Work out the finished part from the listing and answer in its coordinate system (mm). A direction names the side the tool comes from. Coordinates: 2 decimals unless noted, no trailing zeros. Order: outer loops, then holes, each group sorted by start corner. A loop starts at its lowest first (then second) coordinate and runs counter-clockwise, first axis right, second up. Notation, with made-up numbers: M 10,-15 L 26,-15 A23 ccw 26,19 Z; hole C 52,75.25 d3. An arc over 180 degrees is marked long. Answer in a Markdown table with one row per item. Add a question column.
Item 1: The part is cut by section B-B (z = 4). Write down the section's boundary in (x, y).
Item 2: Which of the six approach directions +Z, -Z, +X, -X, +Y, -Y give full straight-line access (tool end or side, diameter ignored) to faces 1 (the face through (-15.54, -11.7, 11.1)), 2 (the face through (0, -36, 3)), 3 (the face through (0, -8, 3))?
Item 3: The part is cut by section D-D (z = 13.25). Write down the section's boundary in (x, y).
Item 4: The mould has two halves that part along Y. Classify faces 4 (the face through (-7, -10.32, 10)), 5 (the face through (-5.881, -9.334, 11.236)), 6 (the face through (2, -15.32, 6)): released by +Y, released by -Y, zero draft, split by the parting line, or undercut.
Item 5: Consider line 1 (Y direction, x = -12.85, z = 11.15); line 2 (Y direction, x = -6.15, z = 4.1); line 3 (Y direction, x = -17.25, z = 14.5). Determine where each line is inside the solid, lowest interval first. Write a range as from..to.
Item 6: The part is cut by section A-A (y = -40.5). Write down the section's boundary in (x, z).
Item 7: Flat-ended cylindrical pins translate along their axes: pin 1 Ø2 at (x, y) = (-6.15, -6.15) entering from -Z; pin 2 Ø1.2 at (x, z) = (2.5, 3.5) entering from +Y; pin 3 Ø2 at (y, z) = (-40.5, 11.15) entering from +X. Find the tip coordinate at first contact, or state that the pin passes through.
Item 8: The part is cut by section C-C (y = -6.15). Write down the section's boundary in (x, z).
from build123d import *

# Parameters (mm, degrees)
ESQUISSE1_W             = 22.3
ESQUISSE1_H             = 43
ESQUISSE1_R             = 2.45
BOSS_EXTRU_1_DEPTH      = 5
BOSS_EXTRU_2_START      = -2.47
ESQUISSE2_R             = 2.45
ESQUISSE2_R_2           = 0.7
BOSS_EXTRU_2_DEPTH      = 2.47
ESQUISSE3_W             = 4
ESQUISSE3_H             = 5
ESQUISSE3_W_2           = 3.94
BOSS_EXTRU_3_DEPTH      = 12.3
ESQUISSE4_R             = 0.7
ENL_V_MAT_EXTRU_1_DEPTH = 52.435201954
BOSS_EXTRU_4_DEPTH      = 2
BOSS_EXTRU_5_DEPTH      = 2
ESQUISSE7_R             = 0.7
BOSS_EXTRU_6_DEPTH      = 4


with BuildPart() as part:
    # Esquisse1 → Boss.-Extru.1 (new body)
    with BuildSketch(Plane.XY):
        with Locations((-11.15, -21.5)):
            Rectangle(ESQUISSE1_W, ESQUISSE1_H)
        with Locations((-6.15, -6.15)):
            Circle(ESQUISSE1_R, mode=Mode.SUBTRACT)
    extrude(amount=BOSS_EXTRU_1_DEPTH)

    # Esquisse2 → Boss.-Extru.2 (add)
    with BuildSketch(Plane.XY.offset(5).offset(BOSS_EXTRU_2_START)):
        with Locations((-6.15, -6.15)):
            Circle(ESQUISSE2_R)
        with Locations((-6.15, -6.15)):
            Circle(ESQUISSE2_R_2, mode=Mode.SUBTRACT)
    extrude(amount=BOSS_EXTRU_2_DEPTH)

    # Esquisse3 → Boss.-Extru.3 (add)
    with BuildSketch(Plane.XY.offset(5)):
        with Locations((-20.3, -40.5)):
            Rectangle(ESQUISSE3_W, ESQUISSE3_H)
        with Locations((-13.54, -40.5)):
            Rectangle(ESQUISSE3_W, ESQUISSE3_H)
        with Locations((-20.3, -12.82)):
            Rectangle(ESQUISSE3_W, ESQUISSE3_H)
        with Locations((-13.57, -12.82)):
            Rectangle(ESQUISSE3_W_2, ESQUISSE3_H)
    extrude(amount=BOSS_EXTRU_3_DEPTH)

    # Esquisse4 → Enlèv. mat.-Extru.1 (cut, through all)
    with BuildSketch(Plane.ZY.offset(22.3)):
        with Locations((11.15, -12.82)):
            Circle(ESQUISSE4_R)
        with Locations((11.15, -40.5)):
            Circle(ESQUISSE4_R)
    extrude(amount=-ENL_V_MAT_EXTRU_1_DEPTH, mode=Mode.SUBTRACT)

    # Esquisse5 → Boss.-Extru.4 (add)
    with BuildSketch(Plane.XZ.offset(43)):
        Polygon((-22.3, 17.3), (-11.54, 17.3), (0, 5), (0, 0), (-22.3, 0), align=None)
    extrude(amount=BOSS_EXTRU_4_DEPTH)

    # Esquisse6 → Boss.-Extru.5 (add)
    with BuildSketch(Plane(origin=(0, -10.32, 0), x_dir=(1, 0, 0), z_dir=(0, 1, 0))):
        Polygon((-22.3, -5), (-22.3, -17.3), (-11.6, -17.3), (0, -5), align=None)
    extrude(amount=BOSS_EXTRU_5_DEPTH)

    # Esquisse7 → Boss.-Extru.6 (add)
    with BuildSketch(Plane(origin=(0, 0, 0), x_dir=(0, 0, -1), z_dir=(1, 0, 0))):
        with BuildLine():
            Line((-11.15, -15.32), (0, -15.32))
            Line((0, -15.32), (0, -27.62))
            Line((0, -27.62), (-11.15, -27.62))
            ThreePointArc((-11.15, -27.62), (-17.3, -21.47), (-11.15, -15.32))
        make_face()
        with Locations(Location((-11.15, -21.47, 0), (0, 0, 90))):
            Circle(ESQUISSE7_R, mode=Mode.SUBTRACT)
    extrude(amount=BOSS_EXTRU_6_DEPTH)


solid = part.part
Reply:
| question | item | result |
|---|---|---|
| 1 | outline | M -22.3,-45 L 0,-45 L 0,-27.62 L 4,-27.62 L 4,-15.32 L 0,-15.32 L 0,0 L -22.3,0 Z; hole C -6.15,-6.15 d1.4 |
| 2 | face 1 | +Z |
| 2 | face 2 | +Z, -Z, +X, -Y |
| 2 | face 3 | +Z, -Z, +X, +Y |
| 3 | outline | M -22.3,-45 L -7.74,-45 L -7.74,-43 L -11.54,-43 L -11.54,-38 L -15.54,-38 L -15.54,-43 L -18.3,-43 L -18.3,-38 L -22.3,-38 Z; M -22.3,-15.32 L -18.3,-15.32 L -18.3,-10.32 L -15.54,-10.32 L -15.54,-15.32 L -11.6,-15.32 L -11.6,-10.32 L -7.78,-10.32 L -7.78,-8.32 L -22.3,-8.32 Z; M 0,-27.25 L 4,-27.25 L 4,-15.69 L 0,-15.69 Z |
| 4 | face 4 | undercut |
| 4 | face 5 | zero draft |
| 4 | face 6 | released by +Y |
| 5 | line 1 | y = -45..-41.2, -39.8..-38, -15.32..-13.52, -12.12..-8.32 |
| 5 | line 2 | y = -45..-6.85, -5.45..0 |
| 5 | line 3 | y = -45..-43, -10.32..-8.32 |
| 6 | outline | M -22.3,0 L 0,0 L 0,5 L -11.54,5 L -11.54,10.45 L -15.54,10.45 L -15.54,5 L -18.3,5 L -18.3,10.45 L -22.3,10.45 Z; M -22.3,11.85 L -18.3,11.85 L -18.3,17.3 L -22.3,17.3 Z; M -15.54,11.85 L -11.54,11.85 L -11.54,17.3 L -15.54,17.3 Z |
| 7 | pin 1 | stops at z = 2.53 |
| 7 | pin 2 | stops at y = -15.32 |
| 7 | pin 3 | stops at x = -11.54 |
| 8 | outline | M -22.3,0 L -8.6,0 L -8.6,2.53 L -6.85,2.53 L -6.85,5 L -22.3,5 Z; M -5.45,2.53 L -3.7,2.53 L -3.7,0 L 0,0 L 0,5 L -5.45,5 Z |
